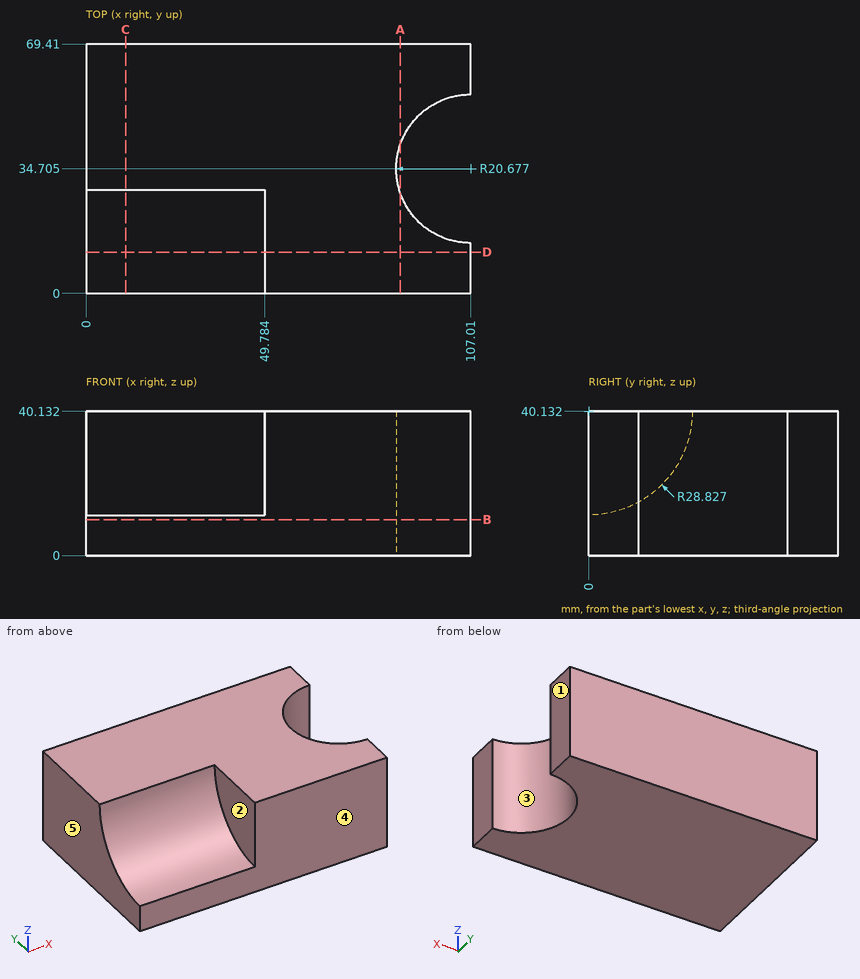
Job drawing, mm, ordinate dimensions from the low corner. One solid piece. A direction names the side the tool comes from. Round coordinates to 2 decimals unless told otherwise and drop trailing zeros. Order: outer loops, then holes, each group sorted by start corner. A loop starts at its lowest first (then second) coordinate and runs counter-clockwise, first axis right, second up. Notation, with made-up numbers: M -10,19.5 L 7,19.5 A15 ccw 7,27.5 Z; hole C -33,-26 d3. An arc over 180 degrees is marked long. Write each question's results on one line, items separated by ' | '. Start each with the question number.
(1) Drop flat-ended pins along their axis: pin 1 (5 mm diameter, centred on y = 50, z = 20.5, fed in from +X); pin 2 (2 mm diameter, centred on y = 36, z = 26, fed in from -X); pin 3 (14.5 mm diameter, centred on y = 10, z = 26.5, fed in from -X); pin 4 (10 mm diameter, centred on y = 30.5, z = 8, fed in from +X) (1 decimal). Give the stop position or say it passes through.
(2) Saw through at C-C, the plane x = 11. Give the cut face in (y, z) (1 decimal), then the cut area to 3 significant figures.
(3) Which spindle directions (+Z, -Z, +X, -X, +Y, -Y) get a long thin tool onto all of the face, cutting with end or side? Do the marked faces 1 and 2. Say none if no direction does.
(4) Probe probe 1 along Y at (x, z) = (95.5, 11); probe 2 along Y at (x, z) = (101, 8); probe 3 along X at (y, z) = (17, 16). List the from-to ranges inside material, lowest first. Write a range as from..to.
(5) Saw through at A-A, the plane x = 87.5. Give the cut face in (y, z).
(6) Saw through at B-B, the plane z = 10. Give the cut face in (x, y) (1 decimal).
(7) Two-plate mould, pull along Y, no slides. Class the marked faces 3, 4 and 5: pulls with the +Y half, pulls with the -Y half, needs draft (parallel to the pull), parting line crosses it, or undercut.
(8) Saw through at D-D, the plane y = 11.5. Give the cut face in (x, z).
Established:
1) pin 1: stops at x = 96.48 | pin 2: stops at x = 0 | pin 3: stops at x = 49.78 | pin 4: stops at x = 88.5
2) outline: M 0,0 L 69.4,0 L 69.4,40.1 L 28.8,40.1 A28.8 cw 0,11.3 Z | area: 2,130 mm^2
3) face 1: +Z, -Z, +X, +Y, -Y | face 2: +Z, -X, -Y
4) probe 1: y = 0..17.53, 51.88..69.41 | probe 2: y = 0..14.92, 54.49..69.41 | probe 3: x = 0..96.33
5) outline: M 0,0 L 27.86,0 L 27.86,40.13 L 0,40.13 Z; M 41.55,0 L 69.41,0 L 69.41,40.13 L 41.55,40.13 Z
6) outline: M 0,0 L 107,0 L 107,14 A20.7 cw 107,55.4 L 107,69.4 L 0,69.4 Z
7) face 3: undercut | face 4: pulls with the -Y half | face 5: needs draft
8) outline: M 0,0 L 107.01,0 L 107.01,40.13 L 49.78,40.13 L 49.78,13.7 L 0,13.7 Z
